from build123d import *

# Parameters (mm, degrees)
SKETCH1_R           = 10
BOSS_EXTRUDE1_DEPTH = 4
SKETCH2_R           = 4
BOSS_EXTRUDE2_DEPTH = 6
SKETCH3_R           = 1.85
CUT_EXTRUDE1_DEPTH  = 18.320508076
SKETCH4_R           = 1.5
CUT_EXTRUDE2_DEPTH  = 16.362291496
CIRPATTERN1_COUNT   = 3


with BuildPart() as part:
    # Sketch1 → Boss-Extrude1 (new body)
    with BuildSketch(Plane(origin=(0, 0, 0), x_dir=(1, 0, 0), z_dir=(0, 1, 0))):
        with Locations(Location((0, 0, 0), (0, 0, 270))):
            Circle(SKETCH1_R)
    extrude(amount=BOSS_EXTRUDE1_DEPTH)

    # Sketch2 → Boss-Extrude2 (add)
    with BuildSketch(Plane(origin=(0, 4, 0), x_dir=(1, 0, 0), z_dir=(0, 1, 0))):
        with Locations(Location((0, 0, 0), (0, 0, 270))):
            Circle(SKETCH2_R)
    extrude(amount=BOSS_EXTRUDE2_DEPTH)

    # Sketch3 → Cut-Extrude1 (cut, through all)
    with BuildSketch(Plane(origin=(0, 10, 0), x_dir=(1, 0, 0), z_dir=(0, 1, 0))):
        with Locations(Location((0, 0, 0), (0, 0, 270))):
            Circle(SKETCH3_R)
    extrude(amount=-CUT_EXTRUDE1_DEPTH, mode=Mode.SUBTRACT)

    # Sketch4 → Cut-Extrude2 (cut, through all)
    with BuildSketch(Plane(origin=(0, 4, 0), x_dir=(1, 0, 0), z_dir=(0, 1, 0))):
        with Locations(Location((0, 7, 0), (0, 0, 270))):
            Circle(SKETCH4_R)
    cut_extrude2 = extrude(amount=-CUT_EXTRUDE2_DEPTH, mode=Mode.SUBTRACT)

    # CirPattern1: Cut-Extrude2 ×3 about axis
    cirpattern1_axis = Axis((0, 0, 0), (0, 1, 0))
    for i in range(1, CIRPATTERN1_COUNT):
        add(cut_extrude2.rotate(cirpattern1_axis, i * 360 / CIRPATTERN1_COUNT), mode=Mode.SUBTRACT)


solid = part.part
The listing builds one solid part. Answer for the finished solid, in the listing's coordinates (mm). Round coordinates to 2 decimals unless told otherwise and drop trailing zeros. Order: outer loops, then holes, each group sorted by start corner. A loop starts at its lowest first (then second) coordinate and runs counter-clockwise, first axis right, second up. Notation, with made-up numbers: (49.25, -24) -> (53.25, -24) arc R9 cw to (53.25, -19) -> close; hole circle Ø4 at (-16.5, -32.5). An arc over 180 degrees is marked (long way). Put each result on its own line as item: value.
Q1. Section C-C, the plane z = 3.5 is taken. Write down the section's boundary in (x, y), and give its area (3 significant figures).
Results list:
outline: (-9.37, 0) -> (-7.56, 0) -> (-7.56, 4) -> (-9.37, 4) -> close; (-4.56, 0) -> (4.56, 0) -> (4.56, 4) -> (1.94, 4) -> (1.94, 10) -> (-1.94, 10) -> (-1.94, 4) -> (-4.56, 4) -> close; (7.56, 0) -> (9.37, 0) -> (9.37, 4) -> (7.56, 4) -> close
area: 74.2 mm^2
Q2. Section B-B, the plane x = 7 is taken. Write down the section's boundary in (y, z).
Results list:
outline: (0, -7.14) -> (4, -7.14) -> (4, 2.33) -> (0, 2.33) -> close; (0, 4.67) -> (4, 4.67) -> (4, 7.14) -> (0, 7.14) -> close
Q3. Determine the mould class of faces 1 (the cylindrical face through (-3.905, 6.958, -0.867)), 2 (the cylindrical face through (0.07, 2.03, -8.5)), 3 (the flat face through (0.1, 4, 4.3)) for opening direction Z: pulls with the +Z half, pulls with the -Z half, needs draft (parallel to the pull), parting line crosses it, or undercut.
Results list:
face 1: parting line crosses it
face 2: undercut
face 3: needs draft
Q4. Each of these flat-tipped pins is pushed along its axis until it touches: P1, Ø4, axis at x = 4, z = 6, coming from the +Y side; P2, Ø5, axis at x = 3.5, z = 6, coming from the -Y side; P3, Ø1.5, axis at y = 8, z = 1, coming from the -X side; P4, Ø3, axis at x = -4, y = 1, coming from the +Z side. Where does it stop, or does it pass through?
Results list:
P1: y = 4
P2: y = 0
P3: x = -3.99
P4: z = 9.68
Q5. Section A-A, the plane z = 0 is taken. Write down the section's boundary in (x, y), and give its area (3 significant figures).
Results list:
outline: (-10, 0) -> (-1.85, 0) -> (-1.85, 10) -> (-4, 10) -> (-4, 4) -> (-10, 4) -> close; (1.85, 0) -> (10, 0) -> (10, 4) -> (4, 4) -> (4, 10) -> (1.85, 10) -> close
area: 91.0 mm^2
Q6. Consider line 1 along X through (y, z) = (2.6, 3.5); line 2 along X through (y, z) = (6, 0); line 3 along X through (y, z) = (3.5, 0). Determine where each line is inside the solid, lowest interval first.
Results list:
line 1: -9.37 to -7.56, -4.56 to 4.56, 7.56 to 9.37
line 2: -4 to -1.85, 1.85 to 4
line 3: -10 to -1.85, 1.85 to 10
Q7. Section D-D, the plane y = 1.75 is taken. Write down the section's boundary in (x, z).
Results list:
outline: circle Ø20 at (0, 0); hole circle Ø3 at (-6.06, 3.5); hole circle Ø3.7 at (0, 0); hole circle Ø3 at (0, -7); hole circle Ø3 at (6.06, 3.5)
